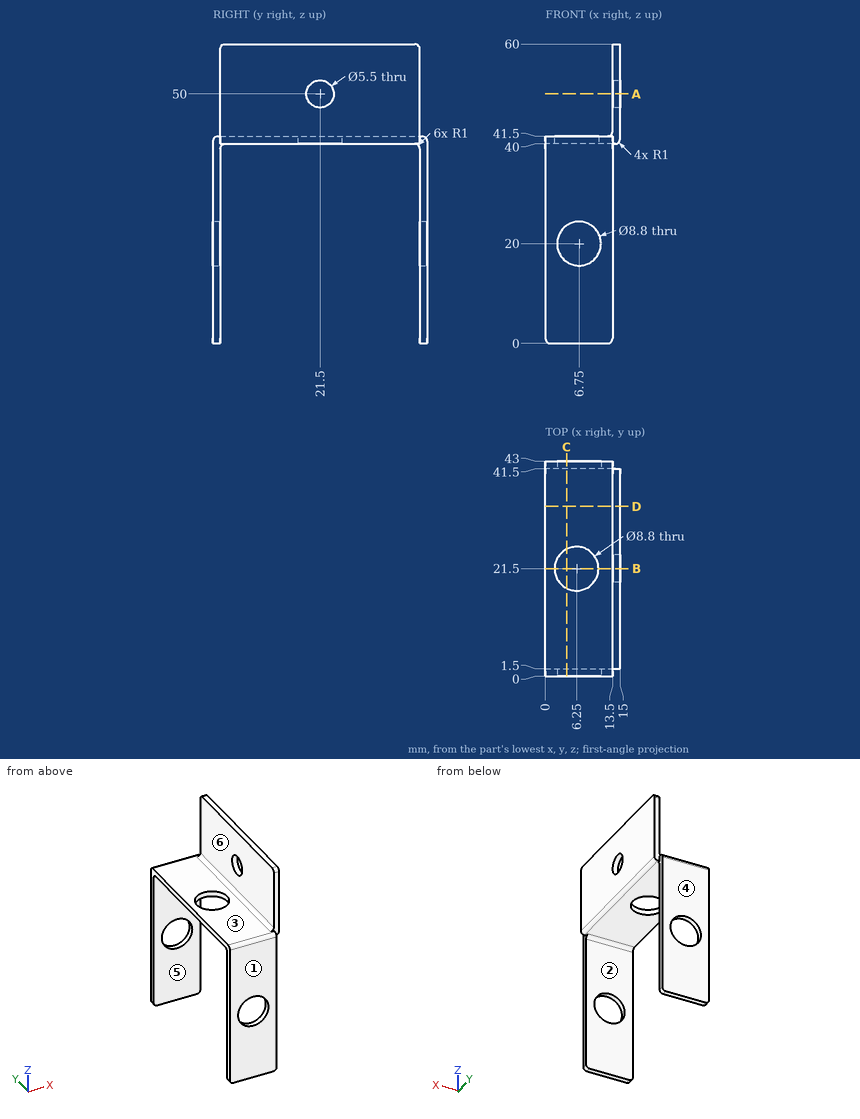
Geometry check sheet. Reference: drawing and pictorial views, mm from the part's lowest x, y, z. A direction names the side the tool comes from. Give positions to 0.01 mm unless a question says otherwise; leave off trailing zeros. Write each loop counter-clockwise with the first axis right and the second up, starting at its lowest first coordinate (ties: lowest second). Pieces come first, ordered by that corner, then holes. Notation, with made-up numbers: (3.25, 83.25) - (34.25, 83.25) arc R31 cw to (34.25, 108.25) - close; hole circle Ø6 at (57.25, 27). An arc over 180 degrees is marked (long way). Put each result on its own line as item: value.
Q1. Scan lines: probe 1 along Y at (x, z) = (1.5, 38); probe 2 along X at (y, z) = (29.5, 56.5); probe 3 along Y at (x, z) = (14.7, 50). Record each from-to range of solid material in increasing order. Write a range as from..to.
Result:
probe 1: 0..1.5, 41.5..43
probe 2: 13.5..15
probe 3: 1.5..18.75, 24.25..41.5
Q2. Section check C-C on x = 4.25. Record the cut outline in (y, z), and give its area (3 significant figures).
Result:
outline: (0, 0) - (1.5, 0) - (1.5, 16.38) - (0, 16.38) - close; (0, 23.62) - (1.5, 23.62) - (1.5, 39) arc R1 cw to (2.5, 40) - (17.58, 40) - (17.58, 41.5) - (1, 41.5) arc R1 ccw to (0, 40.5) - close; (25.42, 40) - (40.5, 40) arc R1 cw to (41.5, 39) - (41.5, 23.62) - (43, 23.62) - (43, 40.5) arc R1 ccw to (42, 41.5) - (25.42, 41.5) - close; (41.5, 0) - (43, 0) - (43, 16.38) - (41.5, 16.38) - close
area: 151 mm2
Q3. Section check B-B on y = 21.5. Record the cut outline in (x, z).
Result:
outline: (0, 40) - (1.85, 40) - (1.85, 41.5) - (0, 41.5) - close; (10.65, 40) - (14, 40) arc R1 ccw to (15, 41) - (15, 47.25) - (13.5, 47.25) - (13.5, 42.5) arc R1 cw to (12.5, 41.5) - (10.65, 41.5) - close; (13.5, 52.75) - (15, 52.75) - (15, 60) - (13.5, 60) - close
Q4. Set-up check for the marked faces 4, 5 and 6: record each of +Z, -Z, +X, -X, +Y, -Y from which the full face is reachable in a straight line by a thin tool's end or side.
Result:
face 4: +Z, -Z, +X, -X, +Y
face 5: -Z, +X, -X
face 6: +Z, -X, +Y, -Y
Q5. Depth check by flat-ended pin: P1, Ø8, axis at x = 3, z = 19, coming from the +Y side; P2, Ø7, axis at x = 6.75, z = 20, coming from the +Y side (3 decimals); P3, Ø0.8, axis at y = 41.5, z = 25.5, coming from the +X side; P4, Ø7, axis at x = 8, y = 17, coming from the -Z side. Enter the tip coordinate at first touch or a pass-through.
Result:
P1: y = 43
P2: through
P3: x = 13.5
P4: z = 40
Q6. Section check A-A on z = 50. Record the cut outline in (x, y), and give its area (4 significant figures).
Result:
outline: (13.5, 1.5) - (15, 1.5) - (15, 18.75) - (13.5, 18.75) - close; (13.5, 24.25) - (15, 24.25) - (15, 41.5) - (13.5, 41.5) - close
area: 51.75 mm2
Q7. Mould release check, pull along Y, two halves, no side actions. Record for the marked faces 1, 2 and 3: released by +Y, released by -Y, zero draft, split by the parting line, or undercut.
Result:
face 1: released by -Y
face 2: undercut
face 3: zero draft
Q8. Section check D-D on y = 34. Record the cut outline in (x, z), and give its area (4 significant figures).
Result:
outline: (0, 40) - (14, 40) arc R1 ccw to (15, 41) - (15, 60) - (13.5, 60) - (13.5, 42.5) arc R1 cw to (12.5, 41.5) - (0, 41.5) - close
area: 50.25 mm2
